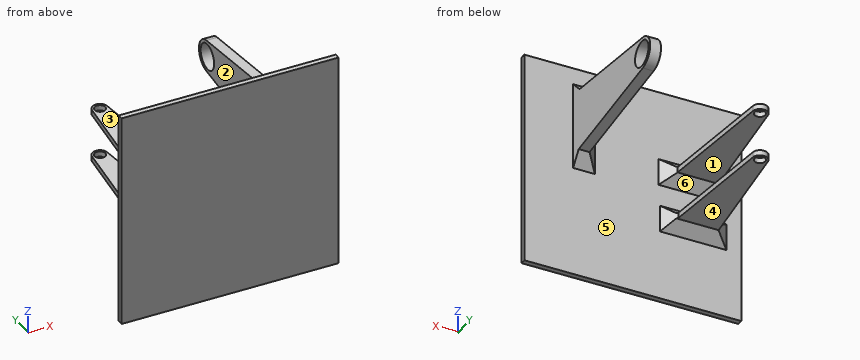
from build123d import *
from OCP.BRepFilletAPI import BRepFilletAPI_MakeChamfer

# Parameters (mm, degrees)
SKETCH_2_W               = 240.549430728
SKETCH_2_H               = 149.540933388
EXTRUDE_1_DEPTH          = 5
SKETCH_6_W               = 93.246571425
SKETCH_6_H               = 149.540933388
EXTRUDE_4_DEPTH          = 5
SKETCH_8_W               = 274.716709757
SKETCH_8_H               = 58.51354913
EXTRUDE_6_DEPTH          = 5
CUT_EXTRUDE_2_DEPTH      = 252.755772101
CUT_EXTRUDE_2_DEPTH_BACK = 252.755772101
SKETCH_9_W               = 59.079292396
SKETCH_9_H               = 149.540933388
SKETCH_10_W              = 104.703380117
SKETCH_10_H              = 208.054482518
CUT_EXTRUDE_3_DEPTH      = 10
SKETCH_12_W              = 200
SKETCH_12_H              = 200
EXTRUDE_7_DEPTH          = 5
SKETCH_13_OUTSIDE_W      = 259.728
SKETCH_13_OUTSIDE_H      = 267.782
SKETCH_13_OUTSIDE_W_2    = 200
SKETCH_13_OUTSIDE_H_2    = 200
CUT_EXTRUDE_4_DEPTH      = 278.64321362
EXTRUDE_START            = -75
SKETCH_18_R              = 5
EXTRUDE_9_DEPTH          = 5
EXTRUDE_START_2          = -45
SKETCH_16_R              = 12
EXTRUDE_10_DEPTH         = 10
CHAMFER_1_SIZE           = 10
CHAMFER_1_SIZE2          = 11.275873044
CHAMFER_1_SIZE2_2        = 11.474527449
CHAMFER_2_SIZE           = 10


with BuildPart() as part:
    # 草图2 → 凸台-拉伸1 (new body)
    with BuildSketch(Plane(origin=(0, 0, 0), x_dir=(1, 0, 0), z_dir=(0, 1, 0))):
        Rectangle(SKETCH_2_W, SKETCH_2_H)
    extrude(amount=EXTRUDE_1_DEPTH)

    # 草图6 → 凸台-拉伸4 (add)
    with BuildSketch(Plane(origin=(0, 5, 0), x_dir=(1, 0, 0), z_dir=(0, 1, 0))):
        with Locations((166.898001077, 0)):
            Rectangle(SKETCH_6_W, SKETCH_6_H)
    extrude(amount=-EXTRUDE_4_DEPTH)

    # 草图8 → 凸台-拉伸6 (add)
    with BuildSketch(Plane(origin=(0, 5, 0), x_dir=(1, 0, 0), z_dir=(0, 1, 0))):
        with Locations((76.162931911, -104.027241259)):
            Rectangle(SKETCH_8_W, SKETCH_8_H)
    extrude(amount=-EXTRUDE_6_DEPTH)

    # 草图9 → 切除-拉伸2 (cut, two sides: drawn at the far end of the back side and taken through both)
    with BuildSketch(Plane(origin=(0, 5, 0), x_dir=(1, 0, 0), z_dir=(0, 1, 0)).offset(-CUT_EXTRUDE_2_DEPTH_BACK)):
        with Locations((-90.735069166, 0)):
            Rectangle(SKETCH_9_W, SKETCH_9_H)
    extrude(amount=CUT_EXTRUDE_2_DEPTH + CUT_EXTRUDE_2_DEPTH_BACK, mode=Mode.SUBTRACT)

    # 草图10 → 切除-拉伸3 (cut)
    with BuildSketch(Plane(origin=(0, 5, 0), x_dir=(1, 0, 0), z_dir=(0, 1, 0))):
        with Locations((-8.84373291, -29.256774565)):
            Rectangle(SKETCH_10_W, SKETCH_10_H)
    extrude(amount=-CUT_EXTRUDE_3_DEPTH, mode=Mode.SUBTRACT)

    # 草图12 → 凸台-拉伸7 (add)
    with BuildSketch(Plane(origin=(0, 5, 0), x_dir=(1, 0, 0), z_dir=(0, 1, 0))):
        with Locations((143.507957149, -25.229533306)):
            Rectangle(SKETCH_12_W, SKETCH_12_H)
    extrude(amount=-EXTRUDE_7_DEPTH)

    # 草图13 outside → 切除-拉伸4 (cut, through all)
    with BuildSketch(Plane(origin=(0, 5, 0), x_dir=(1, 0, 0), z_dir=(0, 1, 0))):
        with Locations((143.508, -29.257)):
            Rectangle(SKETCH_13_OUTSIDE_W, SKETCH_13_OUTSIDE_H)
        with Locations((143.507957149, -25.229533306)):
            Rectangle(SKETCH_13_OUTSIDE_W_2, SKETCH_13_OUTSIDE_H_2, mode=Mode.SUBTRACT)
    extrude(amount=-CUT_EXTRUDE_4_DEPTH, mode=Mode.SUBTRACT)

    # 草图18 → 凸台-拉伸9 (add)
    with BuildSketch(Plane.XY.offset(125.229533306).offset(EXTRUDE_START)):
        with BuildLine():
            Line((108.507957149, 5), (95.467491183, 125.751589006))
            ThreePointArc((95.467491183, 125.751589006), (88.507957149, 132), (81.548423116, 125.751589006))
            Line((81.548423116, 125.751589006), (68.507957149, 5))
            Line((68.507957149, 5), (108.507957149, 5))
        make_face()
        with Locations((88.507957149, 125)):
            Circle(SKETCH_18_R, mode=Mode.SUBTRACT)
    extrude_9 = extrude(amount=-EXTRUDE_9_DEPTH)

    # 镜向1: 凸台-拉伸9 across plane
    add(extrude_9.mirror(Plane.XY.offset(25.229533306)))

    # 草图16 → 凸台-拉伸10 (add)
    with BuildSketch(Plane(origin=(243.507957149, 0, 0), x_dir=(0, 0, -1), z_dir=(1, 0, 0)).offset(EXTRUDE_START_2)):
        with BuildLine():
            Line((-39.779533306, 5), (-54.890001581, 128.817097965))
            ThreePointArc((-54.890001581, 128.817097965), (-69.779533306, 142), (-84.669065031, 128.817097965))
            Line((-84.669065031, 128.817097965), (-99.779533306, 5))
            Line((-99.779533306, 5), (-39.779533306, 5))
        make_face()
        with Locations((-69.779533306, 127)):
            Circle(SKETCH_16_R, mode=Mode.SUBTRACT)
    extrude(amount=-EXTRUDE_10_DEPTH)

    # 倒角1: one chamfer whose edges measure the first distance from different faces: ONE call of the kernel's chamfer builder (chamfer() names one face for all edges)
    chamfer_1_edges_1 = [part.edges().sort_by_distance(p)[0] for p in [
        (88.507957149, 5, 50.229533306),
        (88.507957149, 5, 45.229533306),
        (88.507957149, 5, 5.229533306),
        (88.507957149, 5, 0.229533306),
    ]]
    chamfer_1_edges_2 = [part.edges().sort_by_distance(p)[0] for p in [
        (108.507957149, 5, 47.729533306),
    ]]
    chamfer_1_side_2 = [part.faces().sort_by_distance(p)[0] for p in [
        (101.987724166, 65.375794503, 47.729533306),
    ]]
    chamfer_1_edges_3 = [part.edges().sort_by_distance(p)[0] for p in [
        (68.507957149, 5, 47.729533306),
        (108.507957149, 5, 2.729533306),
    ]]
    chamfer_1_side_3 = [part.faces().sort_by_distance(p)[0] for p in [
        (143.302828944, 5, 24.544148691),
    ]]
    chamfer_1_edges_4 = [part.edges().sort_by_distance(p)[0] for p in [
        (68.507957149, 5, 2.729533306),
    ]]
    chamfer_1_side_4 = [part.faces().sort_by_distance(p)[0] for p in [
        (75.028190132, 65.375794503, 2.729533306),
    ]]
    chamfer_1_edges_5 = [part.edges().sort_by_distance(p)[0] for p in [
        (193.507957149, 5, 39.779533306),
    ]]
    chamfer_1_side_5 = [part.faces().sort_by_distance(p)[0] for p in [
        (193.507957149, 66.908548983, 47.334767443),
    ]]
    chamfer_1_edges_6 = [part.edges().sort_by_distance(p)[0] for p in [
        (193.507957149, 5, 99.779533306),
    ]]
    chamfer_1_side_6 = [part.faces().sort_by_distance(p)[0] for p in [
        (143.302828944, 5, 24.544148691),
    ]]
    chamfer_1 = BRepFilletAPI_MakeChamfer(part.part.solid().wrapped)
    for e in chamfer_1_edges_1:
        chamfer_1.Add(CHAMFER_1_SIZE, e.wrapped)
    for e in chamfer_1_edges_2:
        chamfer_1.Add(CHAMFER_1_SIZE, CHAMFER_1_SIZE2, e.wrapped, chamfer_1_side_2[0].wrapped)  # the first distance lies on this face
    for e in chamfer_1_edges_3:
        chamfer_1.Add(CHAMFER_1_SIZE, CHAMFER_1_SIZE2, e.wrapped, chamfer_1_side_3[0].wrapped)  # the first distance lies on this face
    for e in chamfer_1_edges_4:
        chamfer_1.Add(CHAMFER_1_SIZE, CHAMFER_1_SIZE2, e.wrapped, chamfer_1_side_4[0].wrapped)  # the first distance lies on this face
    for e in chamfer_1_edges_5:
        chamfer_1.Add(CHAMFER_1_SIZE, CHAMFER_1_SIZE2_2, e.wrapped, chamfer_1_side_5[0].wrapped)  # the first distance lies on this face
    for e in chamfer_1_edges_6:
        chamfer_1.Add(CHAMFER_1_SIZE, CHAMFER_1_SIZE2_2, e.wrapped, chamfer_1_side_6[0].wrapped)  # the first distance lies on this face
    add(Compound.cast(chamfer_1.Shape()), mode=Mode.REPLACE)

    # 倒角2
    chamfer_2_edges = [part.edges().sort_by_distance(p)[0] for p in [
        (188.507957149, 5, 69.042269581),
    ]]
    chamfer(chamfer_2_edges, length=CHAMFER_2_SIZE)


solid = part.part
Model file for the job. Use its own axes, mm. Face numbers are marked on the shaded views. A direction names the side the tool comes from. Give positions to 0.01 mm unless a question says otherwise; leave off trailing zeros. Loops run counter-clockwise (first coordinate to the right, second up) from the corner with the lowest first, then second, coordinate; pieces in that order, holes last.
1) Pull direction Z, two halves, no side cores. Call the marked faces 1, 2 and 3: +Z half, -Z half, draft (parallel to the pull), parting line (faces both ways), or undercut.
2) Saw through at A-A (y = 94). Write the cut outline in (x, z).
3) Saw through at B-B (z = -53). Write the cut outline in (x, y).
4) Flat gauge pins, fed straight in: pin 1 Ø5 at (y, z) = (102.5, 56) entering from +X; pin 2 Ø19.5 at (x, y) = (89, 98) entering from +Z; pin 3 Ø9 at (x, y) = (88.51, 125) entering from -Z; pin 4 Ø19.5 at (x, y) = (97, 70.5) entering from -Z. Where does each tip first touch, or does it go through?
5) Saw through at D-D (y = 69). Write the cut outline in (x, z), plus the area to 3 significant figures.
6) Tool access for the marked faces 4, 5 and 6: list every direction of +Z, -Z, +X, -X, +Y, -Y with a clear straight run to the whole face (end or side of a thin tool).
7) Wall check: line 1 (X direction, y = 31, z = 70); line 2 (Y direction, x = 215, z = 29); line 3 (Y direction, x = 102.5, z = -3.5). Give the ranges that are in metal, low to high.
8) Saw through at C-C (x = 102). Write the cut outline in (y, z).
Answer block:
1. face 1: undercut
1. face 2: draft
1. face 3: +Z half
2. outline: (78.12, 0.23) - (98.9, 0.23) - (98.9, 5.23) - (78.12, 5.23) - close; (78.12, 45.23) - (98.9, 45.23) - (98.9, 50.23) - (78.12, 50.23) - close; (188.51, 50.64) - (198.51, 50.64) - (198.51, 88.92) - (188.51, 88.92) - close
3. outline: (43.51, 0) - (243.51, 0) - (243.51, 5) - (43.51, 5) - close
4. pin 1: stops at x = 198.51
4. pin 2: stops at z = 50.23
4. pin 3: passes through
4. pin 4: stops at z = 0.23
5. outline: (75.42, 0.23) - (101.6, 0.23) - (101.6, 5.23) - (75.42, 5.23) - close; (75.42, 45.23) - (101.6, 45.23) - (101.6, 50.23) - (75.42, 50.23) - close; (188.51, 47.59) - (198.51, 47.59) - (198.51, 91.97) - (188.51, 91.97) - close
5. area: 706 mm2
6. face 4: -Z, +X, -X, +Y
6. face 5: +Y
6. face 6: -X, +Y
7. line 1: x = 188.51 to 198.51
7. line 2: y = 0 to 5
7. line 3: y = 0 to 11.27
8. outline: (0, -74.77) - (5, -74.77) - (5, -9.77) - (15, 0.23) - (65.26, 0.23) - (65.26, 5.23) - (15, 5.23) - (5, 15.23) - (5, 35.23) - (15, 45.23) - (65.26, 45.23) - (65.26, 50.23) - (15, 50.23) - (5, 60.23) - (5, 125.23) - (0, 125.23) - close
